```python
from build123d import *

# Parameters (mm, degrees)
F1_DEPTH = 6.35
F2_R     = 2.54


with BuildPart() as f1:
    # F0 (on Front) → F1 (new body, symmetric)
    with BuildSketch(Plane.XZ):
        with BuildLine():
            ThreePointArc((-9.525, 4.7625), (-8.130096, 8.130096), (-4.7625, 9.525))
            Line((-4.7625, 9.525), (0, 9.525))
            Line((0, 9.525), (0, 25.4))
            Line((0, 25.4), (-6.35, 25.4))
            Line((-6.35, 25.4), (-6.35, 14.802732))
            ThreePointArc((-6.35, 14.802732), (-6.841635, 13.105623), (-8.164286, 11.934094))
            ThreePointArc((-8.164286, 11.934094), (-10.37516, 10.37516), (-11.934094, 8.164286))
            ThreePointArc((-11.934094, 8.164286), (-13.105623, 6.841635), (-14.802732, 6.35))
            Line((-14.802732, 6.35), (-25.4, 6.35))
            Line((-25.4, 6.35), (-25.4, 0))
            Line((-25.4, 0), (-9.525, 0))
            Line((-9.525, 0), (-9.525, 4.7625))
        make_face()
    extrude(amount=F1_DEPTH, both=True)

    # F2
    f2_edges = [f1.edges().sort_by_distance(p)[0] for p in [
        (-2.38125, -6.35, 9.525),
        (-8.130096, 6.35, 8.130096),
    ]]
    fillet(f2_edges, radius=F2_R)

    # F3 (on Front) → F4 (revolve, cut)
    with BuildSketch(Plane.XZ):
        Polygon((-20.101366, 0), (-18.513866, 0), (-18.513866, 3.180225), (-16.037366, 6.35), (-13.194864, 9.988236), (-20.101366, 9.988236), align=None)
    revolve(axis=Axis((-20.101366, 0, 3.175), (0, 0, -1)), mode=Mode.SUBTRACT)

    # F5 (on Front) → F6 (revolve, cut)
    with BuildSketch(Plane.XZ):
        Polygon((-9.988236, 13.194864), (-6.35, 16.037366), (-3.180225, 18.513866), (0, 18.513866), (0, 20.101366), (-9.988236, 20.101366), align=None)
    revolve(axis=Axis((-4.994118, 0, 20.101366), (1, 0, 0)), mode=Mode.SUBTRACT)


solid = f1.part
```
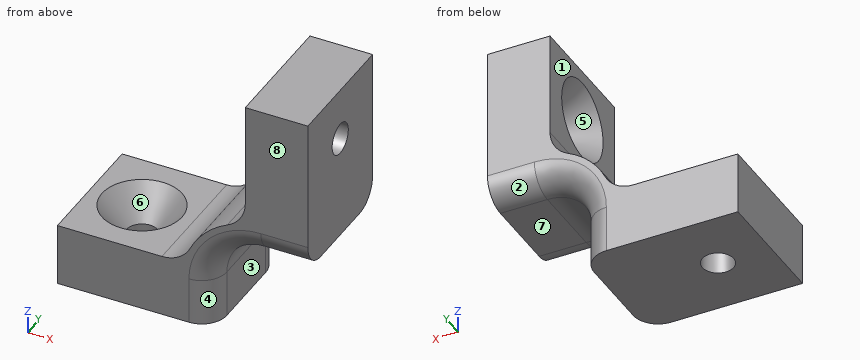
Work out the finished part from the listing and answer in its coordinate system (mm). Face numbers are marked on the shaded views. A direction names the side the tool comes from. Coordinates: 2 decimals unless noted, no trailing zeros. Write each loop counter-clockwise with the first axis right and the second up, starting at its lowest first coordinate (ties: lowest second). Pieces come first, ordered by that corner, then holes. Notation, with made-up numbers: (4.25, 70) - (45.25, 70) arc R24 ccw to (45.25, 93) - close; hole circle Ø4 at (73, 77). An arc over 180 degrees is marked (long way). Answer as a JSON object with one key per item and string values.
Q1. For a pull along Y with two mould halves and no side action, classify the marked faces 5, 6, 7 and 8 as pulls with the +Y half, pulls with the -Y half, needs draft (parallel to the pull), parting line crosses it, or undercut.
Results list:
{"face 5": "undercut", "face 6": "undercut", "face 7": "needs draft", "face 8": "pulls with the -Y half"}
Q2. Given pin 1 Ø6 at (x, y) = (-13.5, -1) entering from -Z; pin 2 Ø5.5 at (x, y) = (-19.5, 2.5) entering from +Z; pin 3 Ø3 at (y, z) = (-1, 19) entering from -X; pin 4 Ø1 at (y, z) = (-2, 18.5) entering from -X, each flat-ended and moving along its own axis, determine where each tip first touches the part or whether it passes through.
Results list:
{"pin 1": "stops at z = 0", "pin 2": "stops at z = 6.35", "pin 3": "stops at x = -4.97", "pin 4": "stops at x = -5.07"}
Q3. Find section A-A (y = 0). State how many separate pieces and enclosed holes the cut face has, plus the area to 3 significant figures.
Results list:
{"separate pieces": "3", "enclosed holes": "0", "area": "169 mm^2"}
Q4. Consider L1, parallel to X at y = 0, z = 0.7 (3 decimals); L2, parallel to X at y = -5.75, z = 17; L3, parallel to Z at x = -6.25, y = 2.75. Determine where each line is inside the solid, lowest interval first. Write a range as from..to.
Results list:
{"L1": "x = -25.4..-21.689, -18.514..-9.525", "L2": "x = -6.35..0", "L3": "z = 9.29..17.22, 22.99..25.4"}
Q5. Which of the six approach directions +Z, -Z, +X, -X, +Y, -Y give full straight-line access (tool end or side, diameter ignored) to the marked faces 1, 2, 3 and 4?
Results list:
{"face 1": "+Z, -X, +Y, -Y", "face 2": "-Z, +X, +Y", "face 3": "-Z, +X, +Y, -Y", "face 4": "-Z, +X, -Y"}
Q6. Find section B-B (x = -12.75). Write down the section's boundary in (y, z).
Results list:
{"outline": "(-6.35, 0) - (6.35, 0) - (6.35, 7.1) - (-6.35, 7.1) - close"}
